The listing builds one solid part. Answer for the finished solid, in the listing's coordinates (mm). Coordinates: 2 decimals unless noted, no trailing zeros. Order: outer loops, then holes, each group sorted by start corner. A loop starts at its lowest first (then second) coordinate and runs counter-clockwise, first axis right, second up.
from build123d import *

# Parameters (mm, degrees)
F0_R     = 5
F0_R_2   = 4.75
F1_DEPTH = 100
F2_R     = 1.5
F2_R_2   = 1.25
F3_DEPTH = 100


with BuildPart() as f1:
    # F0 (on Top) → F1 (new body)
    with BuildSketch(Plane.XY):
        Circle(F0_R)
        Circle(F0_R_2, mode=Mode.SUBTRACT)
    extrude(amount=F1_DEPTH)

    # F2 (on Top) → F3 (join, through all)
    with BuildSketch(Plane.XY):
        with Locations((6.25, 0)):
            Circle(F2_R)
        with Locations((6.25, 0)):
            Circle(F2_R_2, mode=Mode.SUBTRACT)
        with Locations((-6.25, 0)):
            Circle(F2_R)
        with Locations((-6.25, 0)):
            Circle(F2_R_2, mode=Mode.SUBTRACT)
    extrude(amount=F3_DEPTH)


solid = f1.part
(1) Find section A-A on x = -6.25. Determine the outline of the cut face in (y, z).
(2) Find the intervals of material crossed by probe 1 along Y at (x, z) = (0, 79); probe 2 along X at (y, z) = (-0.25, 94); probe 3 along Y at (x, z) = (6.25, 63.5), in increasing order.
(3) Find section B-B on z = 40. Determine the outline of the cut face in (x, y) (3 decimals), then the cut area to 3 significant figures.
(4) Given pin 1 Ø6 at (x, y) = (-1.5, 0) entering from +Z; pin 2 Ø3 at (x, z) = (3.5, 85) entering from +Y; pin 3 Ø2 at (y, z) = (-2, 28.5) entering from +X; pin 4 Ø6 at (x, z) = (-5, 38) entering from -Y, each flat-ended and moving along its own axis, determine where each tip first touches the part or whether it passes through.
(5) Find section C-C on y = -3. Determine the outline of the cut face in (x, z).
Resolved:
1. outline: (-1.5, 0) - (-1.25, 0) - (-1.25, 100) - (-1.5, 100) - close; (1.25, 0) - (1.5, 0) - (1.5, 100) - (1.25, 100) - close
2. probe 1: y = -5 to -4.75, 4.75 to 5
2. probe 2: x = -7.73 to -7.47, -5.03 to -4.74, 4.74 to 5.03, 7.47 to 7.73
2. probe 3: y = -1.5 to -1.25, 1.25 to 1.5
3. outline: (-4.945, -0.74) arc R5 ccw to (4.945, -0.74) arc R1.5 ccw (long way) to (4.945, 0.74) arc R5 ccw to (-4.945, 0.74) arc R1.5 ccw (long way) to start; hole circle Ø2.5 at (-6.25, 0); hole circle Ø9.5 at (0, 0); hole circle Ø2.5 at (6.25, 0)
3. area: 11.5 mm2
4. pin 1: passes through
4. pin 2: stops at y = 4.58
4. pin 3: stops at x = 7.37
4. pin 4: stops at y = -4.58
5. outline: (-4, 0) - (-3.68, 0) - (-3.68, 100) - (-4, 100) - close; (3.68, 0) - (4, 0) - (4, 100) - (3.68, 100) - close
